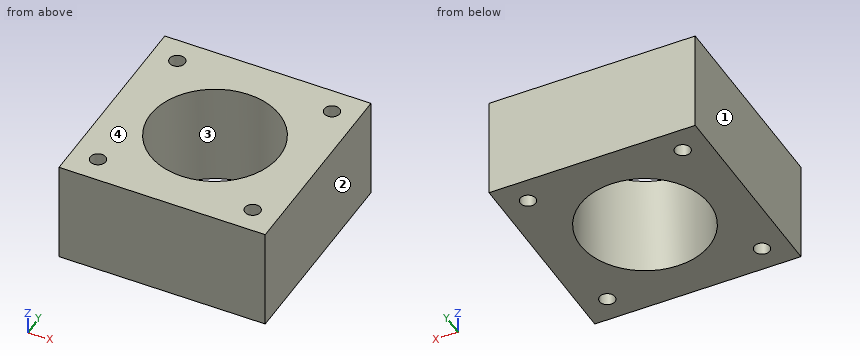
```python
from build123d import *

# Parameters (mm, degrees)
F0_W     = 40
F0_H     = 40
F1_DEPTH = 20
F2_R     = 12.5
F3_DEPTH = 20
F4_R     = 1.5
F5_DEPTH = 25.4


with BuildPart() as f1:
    # F0 (on Top) → F1 (new body)
    with BuildSketch(Plane.XY):
        Rectangle(F0_W, F0_H)
    extrude(amount=F1_DEPTH)

    # F2 (on face) → F3 (cut, through all)
    with BuildSketch(Plane.XY.offset(20)):
        Circle(F2_R)
    extrude(amount=-F3_DEPTH, mode=Mode.SUBTRACT)

    # F4 (on face) → F5 (cut)
    with BuildSketch(Plane.XY.offset(20)):
        with Locations((15, 15)):
            Circle(F4_R)
        with Locations((15, -15)):
            Circle(F4_R)
        with Locations((-15, -15)):
            Circle(F4_R)
        with Locations((-15, 15)):
            Circle(F4_R)
    extrude(amount=-F5_DEPTH, mode=Mode.SUBTRACT)


solid = f1.part
```
Here's how the part is built. I have some questions about the finished solid (model axes, mm). Face numbers are marked on the shaded views. Round coordinates to 2 decimals unless told otherwise and drop trailing zeros. Order: outer loops, then holes, each group sorted by start corner. A loop starts at its lowest first (then second) coordinate and runs counter-clockwise, first axis right, second up. Notation, with made-up numbers: (-7.75, 36.5) -> (13.25, 36.5) arc R7 cw to (13.25, 48.5) -> close; hole circle Ø7 at (18.5, -12.5). An arc over 180 degrees is marked (long way). Use a Markdown table: item, result. Add a question column.
(1) If we mould it in two halves opening along X, with no side actions, what happens to the marked faces 1, 2, 3 and 4? For each: released by +X, released by -X, zero draft, split by the parting line, or undercut.
(2) Suppose I cut it at A-A, the plane y = 15. Please give me the cut outline in (x, z).
(3) Suppose I cut it at C-C, the plane x = 0. Please give me the cut outline in (y, z).
(4) Suppose I cut it at D-D, the plane y = 0.5. Please give me the cut outline in (x, z), and give its area (3 significant figures).
(5) Suppose I cut it at B-B, the plane z = 16. Please give me the cut outline in (x, y), and give its area (3 significant figures).
(6) I need wall thicknesses on line 1 along Y through (x, z) = (-15, 9); line 2 along Y through (x, z) = (0, 12); line 3 along X through (y, z) = (3, 19.25). Which ranges of each line are inside material? Lowest first, please.
Verdict:
| question | item | result |
|---|---|---|
| 1 | face 1 | released by -X |
| 1 | face 2 | released by +X |
| 1 | face 3 | undercut |
| 1 | face 4 | zero draft |
| 2 | outline | (-20, 0) -> (-16.5, 0) -> (-16.5, 20) -> (-20, 20) -> close; (-13.5, 0) -> (13.5, 0) -> (13.5, 20) -> (-13.5, 20) -> close; (16.5, 0) -> (20, 0) -> (20, 20) -> (16.5, 20) -> close |
| 3 | outline | (-20, 0) -> (-12.5, 0) -> (-12.5, 20) -> (-20, 20) -> close; (12.5, 0) -> (20, 0) -> (20, 20) -> (12.5, 20) -> close |
| 4 | outline | (-20, 0) -> (-12.49, 0) -> (-12.49, 20) -> (-20, 20) -> close; (12.49, 0) -> (20, 0) -> (20, 20) -> (12.49, 20) -> close |
| 4 | area | 300 mm2 |
| 5 | outline | (-20, -20) -> (20, -20) -> (20, 20) -> (-20, 20) -> close; hole circle Ø3 at (-15, -15); hole circle Ø3 at (-15, 15); hole circle Ø25 at (0, 0); hole circle Ø3 at (15, -15); hole circle Ø3 at (15, 15) |
| 5 | area | 1,080 mm2 |
| 6 | line 1 | -20 to -16.5, -13.5 to 13.5, 16.5 to 20 |
| 6 | line 2 | -20 to -12.5, 12.5 to 20 |
| 6 | line 3 | -20 to -12.13, 12.13 to 20 |
